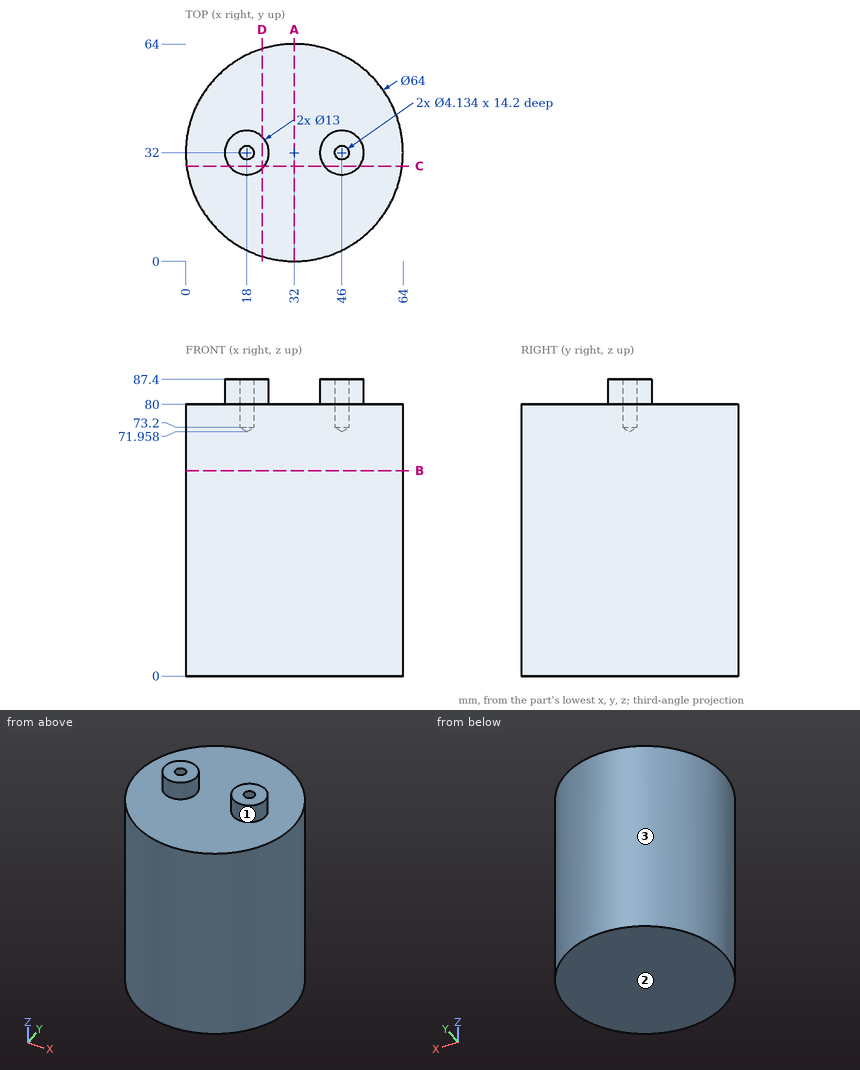
Source: three-view drawing plus pictorial views. Frame: mm from the lowest corner of the part. Give positions to 0.01 mm unless a question says otherwise; leave off trailing zeros. Order: outer loops, then holes, each group sorted by start corner. A loop starts at its lowest first (then second) coordinate and runs counter-clockwise, first axis right, second up. Notation, with made-up numbers: (70, -31.5) - (79, -31.5) arc R20 ccw to (79, -12.5) - close; hole circle Ø2 at (-15.5, 81.25). An arc over 180 degrees is marked (long way). Answer as a JSON object with one key per item and string values. Group by question number.
Q1. Mould query, pull axis X, two halves, no side actions, for the marked faces 1, 2 and 3. Classes: pulls with the +X half, pulls with the -X half, needs draft (parallel to the pull), parting line crosses it, or undercut.
Q2. Cut plane A-A, the plane x = 32. Output: boundary loops of the cut face in (y, z), then the cut area to 3 significant figures.
Q3. First-contact query: pin 1 Ø3 at (x, y) = (47, 40.5) entering from +Z; pin 2 Ø12 at (y, z) = (42.5, 33.5) entering from +X; pin 3 Ø1.5 at (y, z) = (11, 72) entering from -X. Flat tips, straight axial feed; report the tip coordinate or a pass-through.
Q4. Cut plane C-C, the plane y = 28. Output: boundary loops of the cut face in (x, z), then the cut area to 3 significant figures.
Q5. Line query: probe 1 along Z at (x, y) = (28.5, 30); probe 2 along X at (y, z) = (31.5, 35); probe 3 along Y at (x, z) = (46, 76) (3 decimals). Output: solid intervals per line, ascending.
Q6. Cut plane D-D, the plane x = 22.5. Output: boundary loops of the cut face in (y, z).
Q7. Cut plane B-B, the plane z = 60.5. Output: boundary loops of the cut face in (x, y), then the cut area to 3 significant figures.
Results:
{
 "1": {"face 1": "undercut", "face 2": "needs draft", "face 3": "parting line crosses it"},
 "2": {"outline": "(0, 0) - (64, 0) - (64, 80) - (0, 80) - close", "area": "5,120 mm^2"},
 "3": {"pin 1": "z = 80", "pin 2": "x = 63.68", "pin 3": "x = 7.22"},
 "4": {"outline": "(0.25, 0) - (63.75, 0) - (63.75, 80) - (51.12, 80) - (51.12, 87.4) - (40.88, 87.4) - (40.88, 80) - (23.12, 80) - (23.12, 87.4) - (12.88, 87.4) - (12.88, 80) - (0.25, 80) - close", "area": "5,230 mm^2"},
 "5": {"probe 1": "0 to 80", "probe 2": "0 to 64", "probe 3": "3.225 to 29.933, 34.067 to 60.775"},
 "6": {"outline": "(1.44, 0) - (62.56, 0) - (62.56, 80) - (36.69, 80) - (36.69, 87.4) - (27.31, 87.4) - (27.31, 80) - (1.44, 80) - close"},
 "7": {"outline": "circle Ø64 at (32, 32)", "area": "3,220 mm^2"}
}
